from build123d import *


# Not quite as in the source:
# - ends of sketch curves that miss each other by under 0.0002 mm in the source are joined


with BuildPart() as f1:
    # F0 (on Front) → F1 (revolve)
    with BuildSketch(Plane.XZ):
        with BuildLine():
            Line((-7.3999762, -4.999923), (-7.9499112, -4.999876))
            ThreePointArc((-7.9499112, -4.999876), (-8.5406711809, -3.5422157753), (-9.5911861302, -2.3716649112))
            Line((-9.5911861302, -2.3716649112), (-9.4998722, -2.374884))
            Line((-9.4998722, -2.374884), (-9.4998722, 1.625069))
            Line((-9.4998722, 1.625069), (-7.0000502, 1.625069))
            Line((-7.0000502, 1.625069), (-7.0000502, 8.625047))
            Line((-7.0000502, 8.625047), (-10.0000742, 8.625047))
            Line((-10.0000742, 8.625047), (-10.0000742, 14.321571))
            Line((-10.0000742, 14.321571), (-6.5000852, 14.321571))
            Line((-6.5000852, 14.321571), (-5.1849672, 15.080816))
            Line((-5.1849672, 15.080816), (-5.1849672, 21.562471))
            Line((-5.1849672, 21.562471), (-6.5000852, 22.321597))
            Line((-6.5000852, 22.321597), (-10.0000742, 22.321597))
            Line((-10.0000742, 22.321597), (-10.0000742, 25))
            Line((-10.0000742, 25), (-15.0000762, 25))
            Line((-15.0000762, 25), (-15.0000697718, 22.3215925))
            Line((-15.0000697718, 22.3215925), (-15.0000505717, 14.3215729999))
            Line((-15.0000505717, 14.3215729999), (-14.9999562, -25))
            Line((-14.9999562, -25), (4.9999238, -25))
            Line((4.9999238, -25), (14.0001218, -25))
            ThreePointArc((14.0001218, -25), (14.3536028976, -24.8535000977), (14.5000498, -24.499946))
            Line((14.5000498, -24.499946), (14.5000868, -22.999904))
            Line((14.5000868, -22.999904), (15.0000508, -22.999904))
            Line((15.0000508, -22.999904), (15.0000508, -19.719976))
            Line((15.0000508, -19.719976), (14.7301608, -18.099323))
            Line((14.7301608, -18.099323), (13.9495778, -16.653671))
            ThreePointArc((13.9495778, -16.653671), (4.6062496949, -8.3875220734), (-7.3999762, -4.999923))
        make_face()
    revolve(axis=Axis((-15.0000162, 0, 0), (2.4e-06, 0, -1)))


solid = f1.part
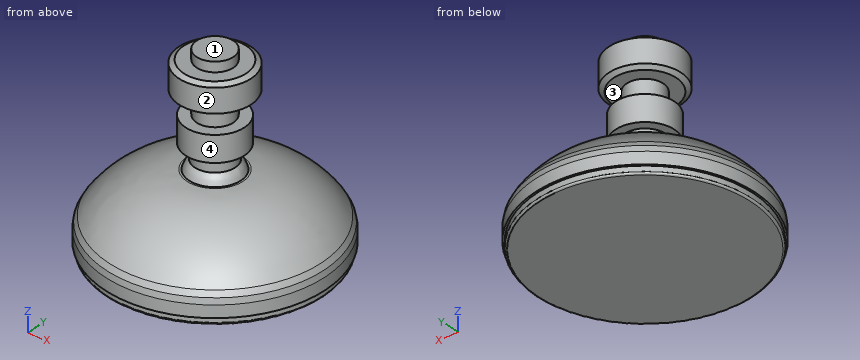
Verification items for the finished model (mm, model axes). Face numbers are marked on the shaded views. Give positions to 0.01 mm unless a question says otherwise; leave off trailing zeros. Write item = value, one per line.
(1) Draft check along Z on the marked faces 1, 2, 3 and 4. Enter one of: released by +Z, released by -Z, zero draft, split by the parting line, or undercut.
Found:
face_1 = released by +Z
face_2 = zero draft
face_3 = undercut
face_4 = undercut
(2) Go/stop test with flat-tipped pins: pin 1 Ø6 at (x, z) = (-19.5, 16.5) entering from +Y; pin 2 Ø5 at (x, z) = (0.5, -19.5) entering from -Y; pin 3 Ø5 at (y, z) = (-1, -8.5) entering from +X. Record where each tip stops, or that it passes through.
Found:
pin_1 = 9.7
pin_2 = -27.03
pin_3 = 8.54
(3) Material ranges on line 1 (Z direction, x = -20, y = 4.5); line 2 (Z direction, x = -9, y = 7.5); line 3 (X direction, y = 2.5, z = 5.5), recorded low to high.
Found:
line_1 = -25 to -4.04, 1.63 to 8.63, 14.32 to 22.32
line_2 = -25 to -5.17, 14.96 to 21.68
line_3 = -22.6 to -7.4
